Autodesk Inventor part; units mm, degrees
ref_plane "YZ Plane" through (0, 0, 0) normal (1, 0, 0) x (0, 1, 0)
ref_plane "XZ Plane" through (0, 0, 0) normal (0, 1, 0) x (-1, 0, 0)
ref_plane "XY Plane" through (0, 0, 0) normal (0, 0, 1) x (1, 0, 0)
sketch "Sketch1" plane through (0, 0, 0) normal (0, 1, 0) x (-1, 0, 0)
  line L0 (0, 0) -> (-40, 0)
  line L1 (-40, 0) -> (-40, 20)
  line L2 (-40, 20) -> (0, 20)
  line L3 (0, 20) -> (0, 0)
  dimension "d0" = 40
  dimension "d1" = 20
revolve "Revolution1" add sketch "Sketch1" angle 360 about axis through (40, 0, 0) along (0, 0, 1)
fillet "Fillet1" radius 15 1 edges at (80, 0, 20)
sketch "Sketch2" plane through (40, 0, 0) normal (0, 0, -1) x (-1, 0, 0)
  circle A0 centre (0, 0) radius 35
  circle A1 centre (0, 0) radius 40
  point P0 (40, 0)
  dimension "d4" = 70
  dimension "d5" = 5
sketch "Sketch3" plane through (40, 0, 0) normal (0, 0, -1) x (-1, 0, 0)
  circle A0 centre (-5, 32.4685) radius 1.5
  circle A1 centre (5, 32.4685) radius 1.5
  point P0 (40, 0)
  point P1 (0, 0)
  dimension "d6" = 3
  dimension "d7" = 3
  dimension "d14" = 10
  dimension "d15" = 5
  dimension "d16" = 5
  dimension "d17" = 32.4685
extrude "Extrusion1" cut sketch "Sketch3" against normal blind 20
sketch "Sketch4" plane through (0, 0, 0) normal (0, 1, 0) x (-1, 0, 0)
  line L0 (-40, 27.46) -> (-40, -52.54) construction
  point P0 (0, 0)
  dimension "d20" = 80
  dimension "d21" = 80
pattern_circular "Circular Pattern1" count 3 over 360 about axis through (40, 0, 27.46) along (0, 0, -1) of "Extrusion1"
equation "\"d6\" = d7"
properties part number "Top_and_Bottom"
Design review of the part built by this model. Coordinates are the model's own, in mm. Give positions to 0.01 mm unless a question says otherwise; leave off trailing zeros. Order: outer loops, then holes, each group sorted by start corner. A loop starts at its lowest first (then second) coordinate and runs counter-clockwise, first axis right, second up. Notation, with made-up numbers: M 58,35.5 L 69,35.5 A26 cw 69,54.5 Z; hole C 31.25,31 d11. An arc over 180 degrees is marked long. One line per question, with ' | ' between items. Start each with the question number.
Q1. We need section A-A (z = 11.5). Write out the cut boundary in (x, y).
Q2. We need section C-C (y = 0). Write out the cut boundary in (x, z).
Q3. The part is to be moulded in two halves that separate along Y. For faces 1 (the face through (45.3, 31, 9.2)), 2 (the face through (1.847, 12.015, 2.465)), 3 (the face through (40, 0, 20)), say which applies: +Y half, -Y half, draft (parallel to the pull), parting line (faces both ways), or undercut.
Q4. We need section B-B (x = 40). Write out the cut boundary in (y, z), plus the area to 3 significant figures.
Q5. For pin 1 Ø4 at (x, y) = (14.38, -20.56) entering from +Z; pin 2 Ø1 at (y, z) = (-8.5, 13) entering from +X; pin 3 Ø8 at (y, z) = (-29, 11.5) entering from +X, all flat-tipped, find the tip position at first contact; note any pin that passes through.
Q6. For L1, parallel to Y at x = 9.5, z = 12; L2, parallel to Y at x = 15, z = 4.5; L3, parallel to Z at x = 15, y = -22.5, list the stretches that pass through material, from the lowest coordinate up. Write a range as [from, to].
Returned:
1) outline: C 40,0 d77.04; hole C 9.38,-11.9 d3; hole C 14.38,-20.56 d3; hole C 35,32.47 d3; hole C 45,32.47 d3; hole C 65.62,-20.56 d3; hole C 70.62,-11.9 d3
2) outline: M 0,0 L 80,0 L 80,5 A15 ccw 65,20 L 15,20 A15 ccw 0,5 Z
3) face 1: undercut | face 2: parting line | face 3: draft
4) outline: M -40,0 L 40,0 L 40,5 A15 ccw 25,20 L -25,20 A15 ccw -40,5 Z | area: 1,500 mm2
5) pin 1: z = 18.81 | pin 2: x = 77.05 | pin 3: x = 69.89
6) L1: [-23.11, -13.4], [-10.41, 23.11] | L2: [-31.22, -21.93], [-19.2, 31.22] | L3: [0, 17.27]
